from build123d import *

# Parameters (mm, degrees)
SKETCH1_W           = 88
SKETCH1_H           = 56
BOSS_EXTRUDE2_DEPTH = 10
SKETCH2_R           = 1.25
CUT_EXTRUDE1_DEPTH  = 10
SKETCH3_W           = 15
SKETCH3_H           = 10
BOSS_EXTRUDE3_DEPTH = 10


with BuildPart() as part:
    # Sketch1 → Boss-Extrude2 (new body)
    with BuildSketch(Plane(origin=(0, 0, 0), x_dir=(1, 0, 0), z_dir=(0, 1, 0))):
        Rectangle(SKETCH1_W, SKETCH1_H)
    extrude(amount=BOSS_EXTRUDE2_DEPTH)

    # Sketch2 → Cut-Extrude1 (cut)
    with BuildSketch(Plane(origin=(0, 10, 0), x_dir=(1, 0, 0), z_dir=(0, 1, 0))):
        with Locations(Location((-40.5, 24.5, 0), (0, 0, 270))):
            Circle(SKETCH2_R)
        with Locations(Location((17.5, 24.5, 0), (0, 0, 270))):
            Circle(SKETCH2_R)
        with Locations(Location((-40.5, -24.5, 0), (0, 0, 270))):
            Circle(SKETCH2_R)
        with Locations(Location((17.5, -24.5, 0), (0, 0, 270))):
            Circle(SKETCH2_R)
    extrude(amount=-CUT_EXTRUDE1_DEPTH, mode=Mode.SUBTRACT)

    # Sketch3 → Boss-Extrude3 (add)
    with BuildSketch(Plane(origin=(0, 10, 0), x_dir=(1, 0, 0), z_dir=(0, 1, 0))):
        with Locations((34, 19)):
            Rectangle(SKETCH3_W, SKETCH3_H)
        with Locations((34, 0)):
            Rectangle(SKETCH3_W, SKETCH3_H)
        with Locations((34, -19)):
            Rectangle(SKETCH3_W, SKETCH3_H)
    extrude(amount=BOSS_EXTRUDE3_DEPTH)


solid = part.part
Verification items for the finished model (mm, model axes). A direction names the side the tool comes from. Coordinates: 2 decimals unless noted, no trailing zeros. Order: outer loops, then holes, each group sorted by start corner. A loop starts at its lowest first (then second) coordinate and runs counter-clockwise, first axis right, second up.
Item 1: Depth check by flat-ended pin: pin 1 (11 mm diameter, centred on y = 16.5, z = -2, fed in from -X); pin 2 (3 mm diameter, centred on x = 36.5, y = 12.5, fed in from -Z); pin 3 (8 mm diameter, centred on y = 16.5, z = 10.5, fed in from +X). Enter the tip coordinate at first touch or a pass-through.
Filled in:
pin 1: stops at x = 26.5
pin 2: stops at z = -24
pin 3: stops at x = 41.5
Item 2: Section check B-B, the plane x = 17.5. Enter the section's corners in (y, z), then the cut area to 3 significant figures.
Filled in:
outline: (0, -28) - (10, -28) - (10, -25.75) - (0, -25.75) - close; (0, -23.25) - (10, -23.25) - (10, 23.25) - (0, 23.25) - close; (0, 25.75) - (10, 25.75) - (10, 28) - (0, 28) - close
area: 510 mm2
Item 3: Release check for a two-part mould opening along X. For faces 1 (the face through (34, 15, -14)), 2 (the face through (17.021, 5.07, -23.345)), 3 (the face through (41.5, 15, 19)) record: +X half, -X half, draft (parallel to the pull), parting line (faces both ways), or undercut.
Filled in:
face 1: draft
face 2: undercut
face 3: +X half
Item 4: Access from +Z, -Z, +X, -X, +Y, -Y to the whole of each face (thin tool, end or side, straight path). Record for faces 4 (the face through (34, 15, 24)), 5 (the face through (34, 15, -5)), 6 (the face through (26.5, 15, 0)).
Filled in:
face 4: +Z, +X, -X, +Y
face 5: +X, -X, +Y
face 6: +Z, -Z, -X, +Y
Item 5: Section check D-D, the plane z = -12. Enter the section's corners in (x, y).
Filled in:
outline: (-44, 0) - (44, 0) - (44, 10) - (-44, 10) - close
Item 6: Section check C-C, the plane z = 0.5. Enter the section's corners in (x, y), then the cut area to 3 significant figures.
Filled in:
outline: (-44, 0) - (44, 0) - (44, 10) - (41.5, 10) - (41.5, 20) - (26.5, 20) - (26.5, 10) - (-44, 10) - close
area: 1,030 mm2
Item 7: Section check A-A, the plane y = 13. Enter the section's corners in (x, z).
Filled in:
outline: (26.5, -24) - (41.5, -24) - (41.5, -14) - (26.5, -14) - close; (26.5, -5) - (41.5, -5) - (41.5, 5) - (26.5, 5) - close; (26.5, 14) - (41.5, 14) - (41.5, 24) - (26.5, 24) - close
Item 8: Material ranges on L1, parallel to X at y = 4.5, z = -24.5; L2, parallel to Y at x = -39, z = 8, recorded low to high.
Filled in:
L1: x = -44 to -41.75, -39.25 to 16.25, 18.75 to 44
L2: y = 0 to 10
